Design review of the part built by this model. Coordinates are the model's own, in mm. Face numbers are marked on the shaded views. Round coordinates to 2 decimals unless told otherwise and drop trailing zeros. Write each loop counter-clockwise with the first axis right and the second up, starting at its lowest first coordinate (ties: lowest second). Pieces come first, ordered by that corner, then holes. Notation, with made-up numbers: (84, -28) - (128, -28) arc R24 ccw to (128, 5) - close; hole circle Ø6 at (70, 87). An arc over 180 degrees is marked (long way). Use one line per item in the form item = value.
```python
from build123d import *

# Parameters (mm, degrees)
F0_W        = 50
F0_H        = 25
F0_W_2      = 46.83
F0_H_2      = 21.83
F1_DEPTH    = 48.08
F2_T1_DEPTH = 178.5841493983
F3_T1_DEPTH = 178.5841493983


# Not quite as in the source:
# - a fillet or chamfer that OpenCascade refuses, or shapes differently, is made with other operations: its cross-section is extruded or revolved along the edge and cut away or added


with BuildPart() as f1:
    # F0 (on Front) → F1 (new body, symmetric)
    with BuildSketch(Plane.XZ):
        Rectangle(F0_W, F0_H)
        Rectangle(F0_W_2, F0_H_2, mode=Mode.SUBTRACT)
    extrude(amount=F1_DEPTH, both=True)

    # F2: chamfer of 25 on 1 edges, made by hand

    # F2_s2 → F2_t1 (cut)
    with BuildSketch(Plane.YZ.offset(-89.2920746991)):
        Polygon((-48.08, 12.5), (-23.08, -12.5), (-48.08, -12.5), align=None)
    extrude(amount=F2_T1_DEPTH, mode=Mode.SUBTRACT)

    # F3: chamfer of 25 on 1 edges, made by hand

    # F3_s2 → F3_t1 (cut)
    with BuildSketch(Plane.YZ.offset(-89.2920746991)):
        Polygon((23.08, -12.5), (48.08, 12.5), (48.08, -12.5), align=None)
    extrude(amount=F3_T1_DEPTH, mode=Mode.SUBTRACT)


solid = f1.part
```
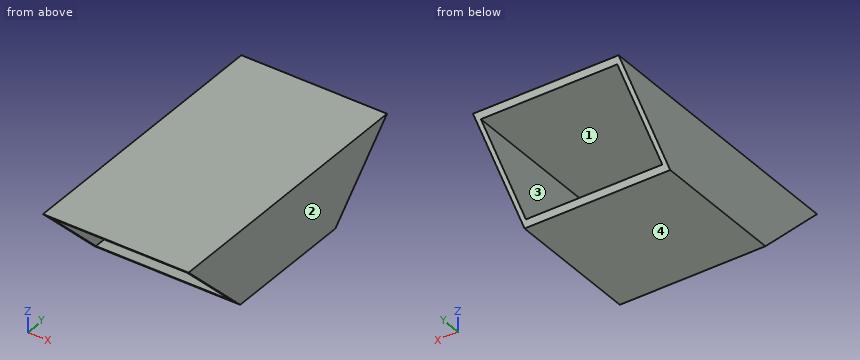
Q1. We need section C-C on x = 20.5. Write out the cut boundary in (y, z) (3 decimals), then the cut area to 3 significant figures.
Calculated:
outline = (-48.08, 12.5) - (-46.495, 10.915) - (46.495, 10.915) - (48.08, 12.5) - close; (-24.665, -10.915) - (-23.08, -12.5) - (23.08, -12.5) - (24.665, -10.915) - close
area = 226 mm2
Q2. For P1, Ø6, axis at x = 9.5, y = 36, coming from the -Z side (3 decimals); P2, Ø8, axis at x = -20, z = -1, coming from the +Y side, all flat-tipped, find the tip position at first contact; note any pin that passes through.
Calculated:
P1 = 10.915
P2 = 36.66
Q3. Draft analysis for pull direction Z (two halves, no side actions). For the marked faces 1, 2, 3 and 4, state which applies: released by +Z, released by -Z, zero draft, split by the parting line, or undercut.
Calculated:
face_1 = undercut
face_2 = zero draft
face_3 = undercut
face_4 = released by -Z
Q4. We need section B-B on y = -11. Write out the cut boundary in (x, z) (3 decimals).
Calculated:
outline = (-25, -12.5) - (25, -12.5) - (25, 12.5) - (-25, 12.5) - close; hole (-23.415, -10.915) - (23.415, -10.915) - (23.415, 10.915) - (-23.415, 10.915) - close
Q5. We need section D-D on y = -31.5. Write out the cut boundary in (x, z) (3 decimals).
Calculated:
outline = (-25, -4.08) - (-23.415, -4.08) - (-23.415, 10.915) - (23.415, 10.915) - (23.415, -4.08) - (25, -4.08) - (25, 12.5) - (-25, 12.5) - close
Q6. To check wall thickness, follow line 1 along X through (y, z) = (20.5, 7.25) (3 decimals); line 2 along Z through (x, y) = (-5.5, 11.5) (3 decimals); line 3 along Z through (x, y) = (2, -30.5) (3 decimals). State the ranges of each line that lie inside material, in increasing order. Write a range as from..to.
Calculated:
line_1 = -25..-23.415, 23.415..25
line_2 = -12.5..-10.915, 10.915..12.5
line_3 = 10.915..12.5
Q7. We need section A-A on z = 9. Write out the cut boundary in (x, y) (3 decimals), then the cut area to 3 significant figures.
Calculated:
outline = (-25, -44.58) - (-23.415, -44.58) - (-23.415, 44.58) - (-25, 44.58) - close; (23.415, -44.58) - (25, -44.58) - (25, 44.58) - (23.415, 44.58) - close
area = 283 mm2
